Autodesk Inventor part; units mm, degrees
ref_plane "YZ Plane" through (0, 0, 0) normal (1, 0, 0) x (0, 1, 0)
ref_plane "XZ Plane" through (0, 0, 0) normal (0, 1, 0) x (-1, 0, 0)
ref_plane "XY Plane" through (0, 0, 0) normal (0, 0, 1) x (1, 0, 0)
sketch "Sketch1" plane through (0, 0, 0) normal (0, 1, 0) x (-1, 0, 0)
  line L0 (0, 0) -> (0, -2.8)
  line L1 (0, -2.8) -> (9.5, -2.8)
  line L2 (0, 0) -> (12.5, 0)
  line L3 (12.5, 0) -> (12.5, -2.8)
  line L4 (9.5, -2.8) -> (9.5, -5.05)
  line L5 (9.5, -5.05) -> (2.5, -5.3)
  line L6 (2.5, -5.3) -> (2.5, -7.3)
  line L7 (12.5, -7.3) -> (12.5, -7.3)
  line L8 (12.5, -7.3) -> (12.5, -2.8)
  line L9 (12.5, -2.8) -> (12.5, -2.8)
  arc A0 (2.5, -7.3) -> (12.5, -7.3) centre (7.5, 0.2833) ccw
  line L10 (14.5304, -7.3) -> (10.3082, -7.3) construction
  dimension "d1" = 2.8
  dimension "d2" = 12.5
  dimension "d3" = 9.5
  dimension "d4" = 3
  dimension "d6" = 4.5
  dimension "d8" = 7.5
  dimension "d9" = 2
  dimension "d13" = 2.25
  dimension "d14" = 10
  dimension "d15" = 1.5
extrude "Extrusion1" add sketch "Sketch1" along normal blind 2.8
properties part number "Cuvette_retainer2"
Work out the finished part from the listing and answer in its coordinate system (mm). A direction names the side the tool comes from. Give positions to 0.01 mm unless a question says otherwise; leave off trailing zeros. Order: outer loops, then holes, each group sorted by start corner. A loop starts at its lowest first (then second) coordinate and runs counter-clockwise, first axis right, second up. Notation, with made-up numbers: (88.5, 21.5) -> (109.5, 21.5) arc R16 cw to (109.5, 47.5) -> close; hole circle Ø4 at (-16.5, 70.5). An arc over 180 degrees is marked (long way). One line per item, written item: value.
Item 1: Find section B-B, the plane y = 0.5. Give the vertices of the cut face in (x, z), plus the area to 3 significant figures.
Answer sheet:
outline: (-12.5, -7.3) arc R9.08 ccw to (-2.5, -7.3) -> (-2.5, -5.3) -> (-9.5, -5.05) -> (-9.5, -2.8) -> (0, -2.8) -> (0, 0) -> (-12.5, 0) -> close
area: 73.6 mm²
Item 2: Flat-ended cylindrical pins translate along their axes: P1, Ø0.6, axis at y = 1.5, z = -6, coming from the +X side; P2, Ø2, axis at x = -3.5, z = -4, coming from the -Y side. Find the tip coordinate at first contact, or state that the pin passes through.
Answer sheet:
P1: x = -2.5
P2: through
Item 3: Find section A-A, the plane x = -3.5. Give the vertices of the cut face in (y, z), plus the area to 3 significant figures.
Answer sheet:
outline: (0, -7.87) -> (2.8, -7.87) -> (2.8, -5.26) -> (0, -5.26) -> close; (0, -2.8) -> (2.8, -2.8) -> (2.8, 0) -> (0, 0) -> close
area: 15.1 mm²
Item 4: A tool of negligible diameter and unlimited length cuts with its end or side. For faces 4 (the flat face through (-2.5, 1, -6)), 5 (the flat face through (-5, 1, -2.8)), 6 (the flat face through (-7.6, 0, -5.3)), from which of +Z, -Z, +X, -X, +Y, -Y can it reach the whole face along a straight path? Write none if from no direction.
Answer sheet:
face 4: -Z, +X, +Y, -Y
face 5: +X, +Y, -Y
face 6: +Z, -Z, +X, -X, -Y
Item 5: Find section C-C, the plane z = -3.75. Give the vertices of the cut face in (x, y).
Answer sheet:
outline: (-12.5, 0) -> (-9.5, 0) -> (-9.5, 2.8) -> (-12.5, 2.8) -> close
Item 6: Find section D-D, the plane x = -1.5. Give the vertices of the cut face in (y, z), plus the area to 3 significant figures.
Answer sheet:
outline: (0, -2.8) -> (2.8, -2.8) -> (2.8, 0) -> (0, 0) -> close
area: 7.84 mm²
Item 7: Straight lines are drawn through the part: probe 1 along X at (y, z) = (0.2, -3.25); probe 2 along X at (y, z) = (1.75, -6.5); probe 3 along Z at (x, y) = (-2, 0.25). For each, find the intervals that lie inside material, in ascending order.
Answer sheet:
probe 1: -12.5 to -9.5
probe 2: -12.5 to -2.5
probe 3: -2.8 to 0
Item 8: Determine the mould class of faces 1 (the flat face through (-12.5, 1, -4)), 2 (the flat face through (-6, 1, 0)), 3 (the flat face through (-9.5, 1, -4)) for opening direction Z: released by +Z, released by -Z, zero draft, split by the parting line, or undercut.
Answer sheet:
face 1: zero draft
face 2: released by +Z
face 3: undercut
